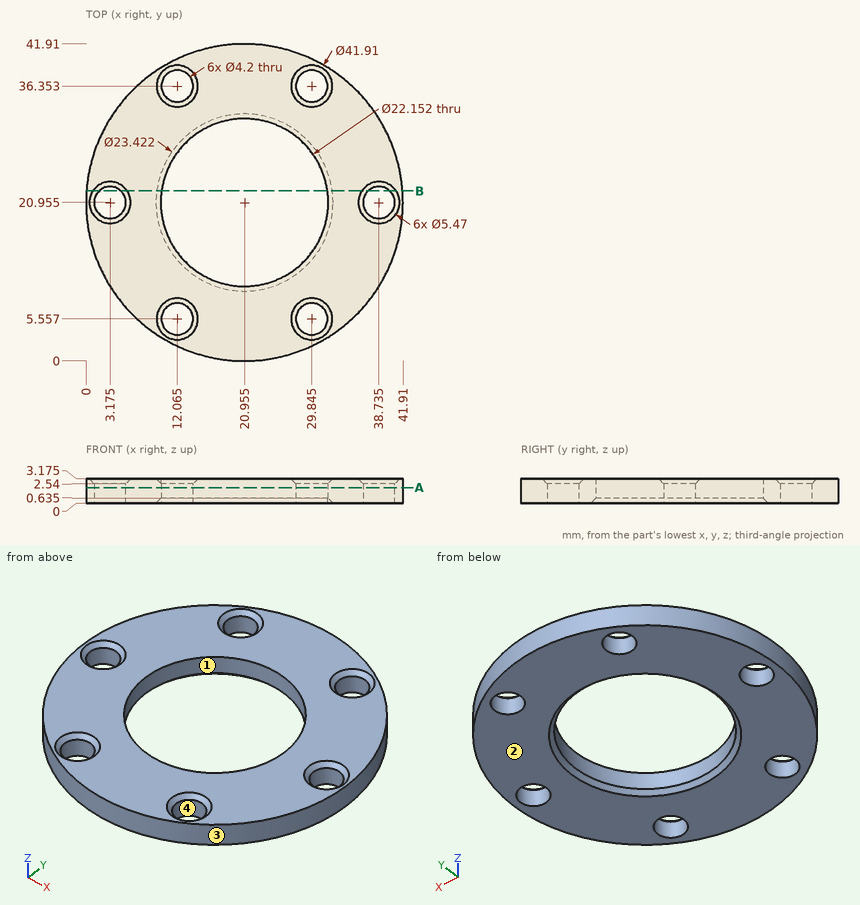
Input: dimensioned drawing with shaded views. Units: mm. Origin: part minimum x, y, z. Give positions to 0.01 mm unless a question says otherwise; leave off trailing zeros. Order: outer loops, then holes, each group sorted by start corner. A loop starts at its lowest first (then second) coordinate and runs counter-clockwise, first axis right, second up.
(1) Section query B-B (y = 22.5). State how many separate pieces and enclosed holes the cut face has, plus the area to 3 significant figures.
(2) Contact query for flat-ended pins moving along their axis: P1, Ø5, axis at x = 12.06, y = 36.35, coming from the +Z side (1 decimal); P2, Ø1, axis at y = 8, z = 1, coming from the +X side. Output: stop coordinate, or through.
(3) Material intervals for line 1 along X through (y, z) = (21, 1.75) (1 decimal); line 2 along Y through (x, z) = (29.5, 0.3) (1 decimal); line 3 along X through (y, z) = (37, 0.35) (1 decimal), sorted ascending.
(4) Pull-direction query (X, two-part tool) for the marked faces 1, 2, 3 and 4; classes: +X half, -X half, draft (parallel to the pull), parting line (faces both ways), or undercut.
(5) Section query A-A (z = 2.05). Return the cut outline in (x, y) (1 decimal), plus the area to 3 significant figures.
Outcome:
1. separate pieces: 4
1. enclosed holes: 0
1. area: 43.5 mm2
2. P1: stops at z = 2.9
2. P2: stops at x = 37.81
3. line 1: x = 0 to 1.1, 5.3 to 9.9, 32 to 36.6, 40.8 to 41.9
3. line 2: y = 1.8 to 3.5, 7.6 to 13.4, 28.5 to 34.3, 38.4 to 40.1
3. line 3: x = 7.5 to 10.1, 14.1 to 27.8, 31.8 to 34.4
4. face 1: undercut
4. face 2: draft
4. face 3: parting line
4. face 4: undercut
5. outline: circle Ø41.9 at (21, 21); hole circle Ø4.2 at (3.2, 21); hole circle Ø22.2 at (21, 21); hole circle Ø4.2 at (12.1, 5.6); hole circle Ø4.2 at (12.1, 36.4); hole circle Ø4.2 at (29.8, 5.6); hole circle Ø4.2 at (29.8, 36.4); hole circle Ø4.2 at (38.7, 21)
5. area: 911 mm2
